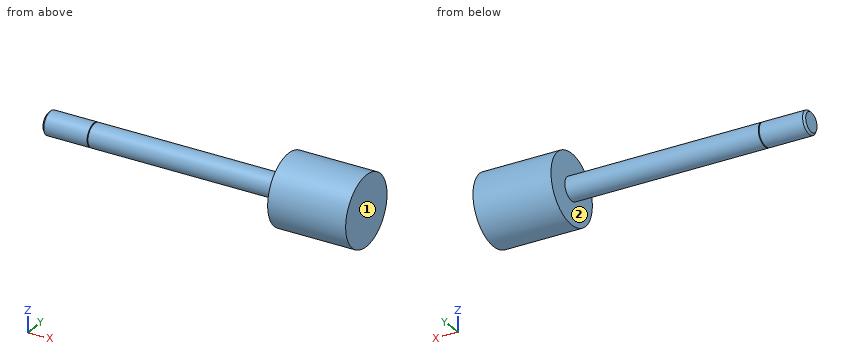
Autodesk Inventor part; units mm, degrees
ref_plane "dia1_XY" through (0, 3.175, 0) normal (1, 0, 0) x (0, 0, -1)
ref_plane "dia1_YZ" through (0, 3.175, 0) normal (0, 0, -1) x (0, 1, 0)
ref_plane "dia1_ZX" through (0, 3.175, 0) normal (0, 1, 0) x (1, 0, 0)
sketch "Sketch_1" plane through (0, 0, 0) normal (0, 0, 1) x (1, 0, 0)
  line L0 (74.6252, 0) -> (0, 0)
  line L1 (0, 0) -> (0, 3.175)
  line L2 (0, 3.175) -> (53.1876, 3.175)
  line L3 (53.1876, 3.175) -> (53.1876, 9.6203)
  line L4 (53.1876, 9.6203) -> (74.6252, 9.6203)
  line L5 (74.6252, 9.6203) -> (74.6252, 0)
  line L6 (74.6252, 0) -> (0, 0)
revolve "Revolution1" add sketch "Sketch_1" angle 360 about axis through (74.6252, 0, 0) along (1, 0, 0)
sketch "Sketch_3" plane through (0, 0, 0) normal (0, 0, 1) x (1, 0, 0)
  line L0 (0, 0) -> (-12.7, 0)
  line L1 (-12.7, 0) -> (-12.7, 2.634)
  line L2 (-12.7, 2.634) -> (-12.159, 3.175)
  line L3 (-12.159, 3.175) -> (0, 3.175)
  line L4 (0, 3.175) -> (0, 0)
  line L5 (0, 0) -> (-12.7, 0)
revolve "Revolution2" add sketch "Sketch_3" angle 360 about axis through (0, 0, 0) along (1, 0, 0)
sketch "Sketch_30" plane through (0, 0, 0) normal (0, 0, 1) x (1, 0, 0)
  line L0 (0, 0) -> (-0.254, 0)
  line L1 (-0.254, 3.429) -> (-0.254, 2.921)
  line L2 (-0.254, 2.921) -> (0, 2.921)
  line L3 (0, 2.921) -> (0, 3.429)
  line L4 (0, 3.429) -> (-0.254, 3.429)
revolve "Revolution3" cut sketch "Sketch_30" angle 360 about axis through (0, 0, 0) along (1, 0, 0)
ref_plane "dia1_XY" through (0, 3.175, 0) normal (1, 0, 0) x (0, 0, -1)
ref_plane "dia1_YZ" through (0, 3.175, 0) normal (0, 0, -1) x (0, 1, 0)
ref_plane "dia1_ZX" through (0, 3.175, 0) normal (0, 1, 0) x (1, 0, 0)
ref_plane "dia12_XY" through (0, 0, 10.9537) normal (1, 0, 0) x (0, 0, -1)
ref_plane "dia12_YZ" through (0, 0, 10.9537) normal (0, 0, -1) x (0, 1, 0)
ref_plane "dia12_ZX" through (0, 0, 10.9537) normal (0, 1, 0) x (1, 0, 0)
ref_plane "dia2_XY" through (0, -3.175, 0) normal (1, 0, 0) x (0, 0, -1)
ref_plane "dia2_YZ" through (0, -3.175, 0) normal (0, 0, -1) x (0, 1, 0)
ref_plane "dia2_ZX" through (0, -3.175, 0) normal (0, 1, 0) x (1, 0, 0)
ref_plane "dia22_XY" through (0, 0, -10.9537) normal (1, 0, 0) x (0, 0, -1)
ref_plane "dia22_YZ" through (0, 0, -10.9537) normal (0, 0, -1) x (0, 1, 0)
ref_plane "dia22_ZX" through (0, 0, -10.9537) normal (0, 1, 0) x (1, 0, 0)
ref_plane "rl1_XY" through (-12.7, 0, 0) normal (1, 0, 0) x (0, 0, -1)
ref_plane "rl1_YZ" through (-12.7, 0, 0) normal (0, 0, -1) x (0, 1, 0)
ref_plane "rl1_ZX" through (-12.7, 0, 0) normal (0, 1, 0) x (1, 0, 0)
ref_plane "rl2_XY" through (0, 0, 0) normal (1, 0, 0) x (0, 0, -1)
ref_plane "rl2_YZ" through (0, 0, 0) normal (0, 0, -1) x (0, 1, 0)
ref_plane "rl2_ZX" through (0, 0, 0) normal (0, 1, 0) x (1, 0, 0)
ref_plane "rod_cp_XY" through (0, 0, 0) normal (1, 0, 0) x (0, 0, -1)
ref_plane "rod_cp_YZ" through (0, 0, 0) normal (0, 0, -1) x (0, 1, 0)
ref_plane "rod_cp_ZX" through (0, 0, 0) normal (0, 1, 0) x (1, 0, 0)
ref_plane "thd1_XY" through (-12.7, 3.175, 0) normal (1, 0, 0) x (0, 0, -1)
ref_plane "thd1_YZ" through (-12.7, 3.175, 0) normal (0, 0, -1) x (0, 1, 0)
ref_plane "thd1_ZX" through (-12.7, 3.175, 0) normal (0, 1, 0) x (1, 0, 0)
ref_plane "thd2_XY" through (-12.7, -3.175, 0) normal (1, 0, 0) x (0, 0, -1)
ref_plane "thd2_YZ" through (-12.7, -3.175, 0) normal (0, 0, -1) x (0, 1, 0)
ref_plane "thd2_ZX" through (-12.7, -3.175, 0) normal (0, 1, 0) x (1, 0, 0)
ref_plane "to_rod_clevis_XY" through (-16.764, 0, 0) normal (1, 0, 0) x (0, 0, -1)
ref_plane "to_rod_clevis_YZ" through (-16.764, 0, 0) normal (0, 0, -1) x (0, 1, 0)
ref_plane "to_rod_clevis_ZX" through (-16.764, 0, 0) normal (0, 1, 0) x (1, 0, 0)
properties part number "C-040.5-DP0_rod"
Geometry: final body of the model. Coordinates: model frame, mm. Face numbers are marked on the shaded views. A direction names the side the tool comes from. Coordinates: 2 decimals unless noted, no trailing zeros. Loops run counter-clockwise (first coordinate to the right, second up) from the corner with the lowest first, then second, coordinate; pieces in that order, holes last. Notation, with made-up numbers: (50.5, 2) - (89.5, 2) arc R35 ccw to (89.5, 41) - close; hole circle Ø5 at (79, -2.75). An arc over 180 degrees is marked (long way). Put each result on its own line as item: value. Start each with the question number.
Q1. Pin query (flat end, axial travel): pin 1 Ø6 at (x, y) = (26, 7) entering from +Z; pin 2 Ø8 at (x, z) = (34.5, 5) entering from -Y; pin 3 Ø5 at (x, y) = (26, -2.5) entering from +Z (3 decimals); pin 4 Ø1.5 at (x, y) = (34.5, 3.5) entering from -Z. Return the tip coordinate at first contact, or that it passes through.
Q2. Cut plane C-C, the plane x = 31. Return loops of the section in (y, z) (3 decimals), and give its area (3 significant figures).
Q3. Cut plane A-A, the plane z = 0. Return loops of the section in (x, y) (3 decimals).
Q4. Cut plane D-D, the plane x = 67.5. Return loops of the section in (y, z).
Q5. Line query: line 1 (X direction, y = 2.25, z = 7.5); line 2 (Z direction, x = 32.5, y = 0) (3 decimals); line 3 (Z direction, x = 16.5, y = -1.25). Output: solid intervals per line, ascending.
Q6. Set-up query: the marked faces 1 and 2. Return all of +Z, -Z, +X, -X, +Y, -Y with unobstructed straight access to the full face (end or side cutting, diameter ignored); none if empty.
Filled sheet:
1. pin 1: through
1. pin 2: y = -3.01
1. pin 3: z = 3.175
1. pin 4: z = -1.59
2. outline: circle Ø6.35 at (0, 0)
2. area: 31.7 mm²
3. outline: (-12.7, -2.634) - (-12.159, -3.175) - (-0.254, -3.175) - (-0.254, -2.921) - (0, -2.921) - (0, -3.175) - (53.188, -3.175) - (53.188, -9.62) - (74.625, -9.62) - (74.625, 9.62) - (53.188, 9.62) - (53.188, 3.175) - (0, 3.175) - (0, 2.921) - (-0.254, 2.921) - (-0.254, 3.175) - (-12.159, 3.175) - (-12.7, 2.634) - close
4. outline: circle Ø19.24 at (0, 0)
5. line 1: 53.19 to 74.63
5. line 2: -3.175 to 3.175
5. line 3: -2.92 to 2.92
6. face 1: +Z, -Z, +X, +Y, -Y
6. face 2: -X
